Source: CAD feature listing. Evaluate the final solid. Frame: model axes, mm. Face numbers are marked on the shaded views. A direction names the side the tool comes from. Round coordinates to 2 decimals unless told otherwise and drop trailing zeros. Write each loop counter-clockwise with the first axis right and the second up, starting at its lowest first coordinate (ties: lowest second). Pieces come first, ordered by that corner, then holes. Notation, with made-up numbers: (-37.75, 54.25) -> (-25.75, 54.25) arc R32 cw to (-25.75, 90.25) -> close; hole circle Ø3 at (-25, 55.5). An arc over 180 degrees is marked (long way). Put each result on its own line as item: value.
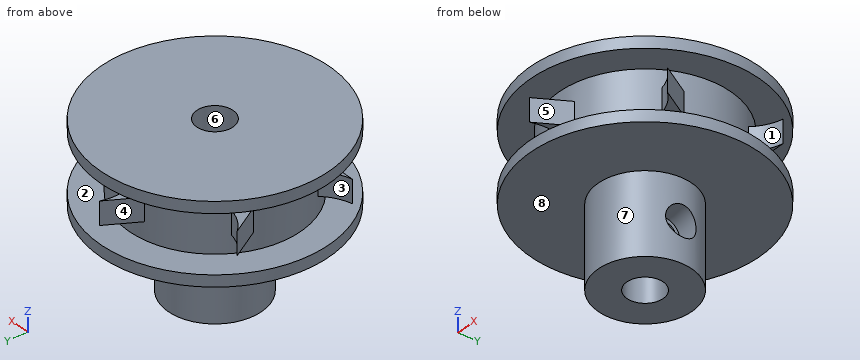
Autodesk Inventor part; units mm, degrees
ref_plane "Work Plane1" through (0, 0, 7) normal (0, 0, -1) x (-1, 0, 0)
ref_plane "Work Plane2" through (8.175, 0, 0) normal (1, 0, 0) x (0, 1, 0)
ref_plane "XZ Plane" through (0, 0, 0) normal (0, 1, 0) x (-1, 0, 0)
sketch "Sketch1" plane through (0, 0, 0) normal (0, 0, 1) x (1, 0, 0)
  circle A0 centre (0, 0) radius 15
  circle A1 centre (0, 0) radius 20
  circle A2 centre (0, 0) radius 3.175
  circle A3 centre (0, 0) radius 8.175
  dimension "d18" = 6.35
  dimension "d19" = 16.35
  dimension "d40" = 30
  dimension "d41" = 5
extrude "Extrusion1" add sketch "Sketch1" along normal blind 14 contours A0 | A2 | A3
extrude "Extrusion2" add sketch "Sketch1" along normal blind 2 contours A1
sketch "Sketch2" plane through (0, 0, 14) normal (0, 0, 1) x (1, 0, 0)
  circle A0 centre (0, 0) radius 15
  circle A1 centre (0, 0) radius 20
extrude "Extrusion3" add sketch "Sketch2" against normal blind 2
ref_plane "Work Plane1" through (0, 0, 7) normal (0, 0, -1) x (-1, 0, 0)
extrude "Extrusion5" cut sketch "Sketch1" along normal up to surface (14 mm away) contours A2
extrude "Extrusion6" add sketch "Sketch1" against normal blind 14 contours A3
ref_plane "Work Plane2" through (8.175, 0, 0) normal (1, 0, 0) x (0, 1, 0)
sketch "Sketch9" plane through (0, 0, 7) normal (0, 0, -1) x (-1, 0, 0)
  circle A0 centre (0, 0) radius 15
  line L0 (0, -15) -> (0, -20) construction
  circle A1 centre (0, 0) radius 20
  arc A2 (0, -15) -> (0, -20) centre (7.5993, -17.5) ccw
  line L1 (0, -20) -> (-3.0701, -14.6825)
  circle A3 centre (0, 0) radius 15
  line L2 (12.9904, -7.5) -> (17.3205, -10) construction
  line L3 (17.3205, -10) -> (11.1803, -10)
  arc A4 (12.9904, -7.5) -> (17.3205, -10) centre (18.9551, -2.1688) ccw
  line L4 (12.9904, 7.5) -> (17.3205, 10) construction
  line L5 (17.3205, 10) -> (14.2504, 4.6825)
  arc A5 (12.9904, 7.5) -> (17.3205, 10) centre (11.3558, 15.3312) ccw
  line L6 (0, 15) -> (0, 20) construction
  line L7 (0, 20) -> (3.0701, 14.6825)
  arc A6 (0, 15) -> (0, 20) centre (-7.5993, 17.5) ccw
  line L8 (-12.9904, 7.5) -> (-17.3205, 10) construction
  line L9 (-17.3205, 10) -> (-11.1803, 10)
  arc A7 (-12.9904, 7.5) -> (-17.3205, 10) centre (-18.9551, 2.1688) ccw
  line L10 (-12.9904, -7.5) -> (-17.3205, -10) construction
  line L11 (-17.3205, -10) -> (-14.2504, -4.6825)
  arc A8 (-12.9904, -7.5) -> (-17.3205, -10) centre (-11.3558, -15.3312) ccw
  point P0 (0, -17.5)
  point P1 (15.1554, -8.75)
  point P2 (15.1554, 8.75)
  point P3 (0, 17.5)
  point P4 (-15.1554, 8.75)
  point P5 (-15.1554, -8.75)
  dimension "d58" = 8
  dimension "d59" = 30
  dimension "d62" = 360
extrude "Extrusion9" add sketch "Sketch9" along normal mid plane 4 contours A0 A5 L5 | A4 L3 A0 | A0 A6 L7 | A2 L1 A0 | L9 A0 A7 | L11 A0 A8
sketch "Sketch10" plane through (8.175, 0, 0) normal (1, 0, 0) x (0, 1, 0)
  line L0 (0, 0) -> (0, -14) construction
  line L1 (3.175, -14) -> (-3.175, -14) construction
  circle A0 centre (0, -7) radius 2.6543
  circle A1 centre (0, -7) radius 2.5273
  dimension "d67" = 5.3086
  dimension "d68" = 5.0546
extrude "Extrusion10" cut sketch "Sketch10" against normal blind 3.81 contours A1
loft "Loft1" cut profiles "Sketch10" section 2 edges at (4.365, -2.5273, -7) contours A0 | A1
hole "Hole2" at (8.175, 0, -7) direction (-1, 0, 0) diameter 3.797 end up to surface
properties part number "leverSpindle"
Q1. Cut plane C-C on x = 5. Output: boundary loops of the cut face in (y, z), and give its area (3 significant figures).
Ans:
outline: (-19.36, 0) -> (-6.47, 0) -> (-6.47, -14) -> (6.47, -14) -> (6.47, 0) -> (19.36, 0) -> (19.36, 2) -> (14.14, 2) -> (14.14, 12) -> (19.36, 12) -> (19.36, 14) -> (-19.36, 14) -> (-19.36, 12) -> (-14.14, 12) -> (-14.14, 2) -> (-19.36, 2) -> close; hole circle Ø5.1 at (0, -7)
area: 598 mm^2
Q2. Reachability of the marked faces 1, 2, 3 and 4 from +Z, -Z, +X, -X, +Y, -Y: full face, straight path, thin tool, end or side. Return the list, or none.
Ans:
face 1: +X
face 2: none
face 3: -X
face 4: -X, +Y
Q3. Cut plane B-B on y = 9. Output: boundary loops of the cut face in (x, z).
Ans:
outline: (-17.86, 0) -> (17.86, 0) -> (17.86, 2) -> (12, 2) -> (12, 5) -> (14.79, 5) -> (14.79, 9) -> (12, 9) -> (12, 12) -> (17.86, 12) -> (17.86, 14) -> (-17.86, 14) -> (-17.86, 12) -> (-12, 12) -> (-12, 2) -> (-17.86, 2) -> close; (-16.74, 5) -> (-16.25, 5) -> (-16.25, 9) -> (-16.74, 9) -> close
Q4. Cut plane D-D on x = -4. Output: boundary loops of the cut face in (y, z), and give its area (3 significant figures).
Ans:
outline: (-19.6, 0) -> (-7.13, 0) -> (-7.13, -14) -> (7.13, -14) -> (7.13, 0) -> (19.6, 0) -> (19.6, 2) -> (14.46, 2) -> (14.46, 12) -> (19.6, 12) -> (19.6, 14) -> (-19.6, 14) -> (-19.6, 12) -> (-14.46, 12) -> (-14.46, 2) -> (-19.6, 2) -> close
area: 646 mm^2
Q5. Material intervals for line 1 (Z direction, x = 16.5, y = 4.5); line 2 (Z direction, x = 3.7, y = 0); line 3 (Y direction, x = 3.25, z = -7), sorted ascending. Write a range as [from, to].
Ans:
line 1: z = [0, 2], [12, 14]
line 2: z = [-14, -8.9], [-5.1, 14]
line 3: y = [-7.5, -1.9], [1.9, 7.5]
Q6. Draft query along Y for the marked faces 5, 6, 7 and 8. Return one class per face: +Y half, -Y half, draft (parallel to the pull), parting line (faces both ways), or undercut.
Ans:
face 5: -Y half
face 6: undercut
face 7: parting line
face 8: draft
Q7. Cut plane A-A on y = 0. Output: boundary loops of the cut face in (x, z) (1 decimal).
Ans:
outline: (-20, 0) -> (-8.2, 0) -> (-8.2, -14) -> (-3.2, -14) -> (-3.2, 14) -> (-20, 14) -> (-20, 12) -> (-15, 12) -> (-15, 2) -> (-20, 2) -> close; (3.2, -14) -> (8.2, -14) -> (8.2, -9.7) -> (4.4, -9.5) -> (4.4, -8.9) -> (3.2, -8.9) -> close; (3.2, -5.1) -> (4.4, -5.1) -> (4.4, -4.5) -> (8.2, -4.3) -> (8.2, 0) -> (20, 0) -> (20, 2) -> (15, 2) -> (15, 12) -> (20, 12) -> (20, 14) -> (3.2, 14) -> close
Q8. Pin query (flat end, axial travel): pin 1 (10 mm diameter, centred on y = -4, z = 2.5, fed in from +X); pin 2 (1.3 mm diameter, centred on x = 13.5, y = 9, fed in from -Z); pin 3 (3.5 mm diameter, centred on y = 0, z = -7, fed in from +X); pin 4 (5 mm diameter, centred on x = -1, z = 2.5, fed in from -Y). Return the tip coordinate at first contact, or that it passes through.
Ans:
pin 1: stops at x = 20
pin 2: stops at z = 0
pin 3: stops at x = -2.65
pin 4: stops at y = -20
